The model under review builds one solid part; all positions refer to its coordinate system, in mm. A direction names the side the tool comes from. Give positions to 0.01 mm unless a question says otherwise; leave off trailing zeros. Write each loop counter-clockwise with the first axis right and the second up, starting at its lowest first coordinate (ties: lowest second). Pieces come first, ordered by that corner, then holes. Notation, with made-up numbers: (55.5, -1) -> (79.5, -1) arc R10 ccw to (79.5, 8) -> close; hole circle Ø4 at (-38.5, 20.5). An arc over 180 degrees is marked (long way). Use CSV: the item, a comma, the result in double quotes.
```python
from build123d import *

# Parameters (mm, degrees)
EXTRUDE_1_DEPTH = 5
SKETCH_2_R      = 11.25
EXTRUDE_2_DEPTH = 2
CHAMFER_1_SIZE  = 1.5
SKETCH_3_W      = 9.552486588
SKETCH_3_H      = 17
EXTRUDE_3_DEPTH = 9
FILLET_1_R      = 1
EXTRUDE_4_DEPTH = 2


with BuildPart() as part:
    # Эскиз1 → Бобышка-Вытянуть1 (new body)
    with BuildSketch(Plane(origin=(0, 0, 0), x_dir=(1, 0, 0), z_dir=(0, 1, 0))):
        with BuildLine():
            Line((-10.75, 1), (-9.698582371, 1))
            ThreePointArc((-9.698582371, 1), (9.75, 0), (-9.698582371, -1))
            Line((-9.698582371, -1), (-10.75, -1))
            Line((-10.75, -1), (-10.75, 1))
        make_face()
    extrude(amount=EXTRUDE_1_DEPTH)

    # Эскиз2 → Бобышка-Вытянуть2 (add)
    with BuildSketch(Plane(origin=(0, 5, 0), x_dir=(1, 0, 0), z_dir=(0, 1, 0))):
        Circle(SKETCH_2_R)
    extrude(amount=EXTRUDE_2_DEPTH)

    # Фаска1
    chamfer_1_edges = [part.edges().sort_by_distance(p)[0] for p in [
        (-11.25, 7, 0),
    ]]
    chamfer(chamfer_1_edges, length=CHAMFER_1_SIZE)

    # Эскиз3 → Бобышка-Вытянуть3 (add)
    with BuildSketch(Plane.XZ):
        Rectangle(SKETCH_3_W, SKETCH_3_H)
    extrude(amount=EXTRUDE_3_DEPTH)

    # Скругление1
    fillet_1_edges = [part.edges().sort_by_distance(p)[0] for p in [
        (-4.776243294, -4.5, 8.5),
        (-4.776243294, -4.5, -8.5),
        (4.776243294, -4.5, -8.5),
        (4.776243294, -4.5, 8.5),
    ]]
    fillet(fillet_1_edges, radius=FILLET_1_R)

    # Эскиз4 → Бобышка-Вытянуть4 (add, symmetric)
    with BuildSketch(Plane(origin=(0, 0, 0), x_dir=(0, 0, -1), z_dir=(1, 0, 0))):
        Polygon((-8.5, -9), (-13.010373574, 1.032772808), (-10.70938382, 4.9), (-9.85, 4.388668944), (-11.885037306, 0.968422681), (-7.587929745, -8.589966039), align=None)
        Polygon((11.885037306, 0.968422681), (7.587929745, -8.589966039), (8.5, -9), (13.010373574, 1.032772808), (10.70938382, 4.9), (9.85, 4.388668944), align=None)
    extrude(amount=EXTRUDE_4_DEPTH, both=True)


solid = part.part
```
Q1. To check wall thickness, follow probe 1 along Z at (x, y) = (1.5, 0.75); probe 2 along Z at (x, y) = (-3.25, -0.75); probe 3 along Y at (x, z) = (6, -6). State the ranges of each line that lie inside material, in increasing order.
Derived:
probe 1,"z = -12.88 to -11.79, -9.63 to 9.63, 11.79 to 12.88"
probe 2,"z = -8.5 to 8.5"
probe 3,"y = 0 to 7"
Q2. Consider section C-C (x = 0). Write out the cut boundary in (y, z), then the cut area to 3 significant figures.
Derived:
outline,"(-9, -8.5) -> (1.03, -13.01) -> (4.9, -10.71) -> (4.39, -9.85) -> (0.97, -11.89) -> (-6.56, -8.5) -> (0, -8.5) -> (0, -9.75) -> (5, -9.75) -> (5, -11.25) -> (5.5, -11.25) -> (7, -9.75) -> (7, 9.75) -> (5.5, 11.25) -> (5, 11.25) -> (5, 9.75) -> (0, 9.75) -> (0, 8.5) -> (-6.56, 8.5) -> (0.97, 11.89) -> (4.39, 9.85) -> (4.9, 10.71) -> (1.03, 13.01) -> (-9, 8.5) -> close"
area,"321 mm2"
Q3. Consider section B-B (y = 4). Write out the cut boundary in (x, z).
Derived:
outline,"(-10.75, -1) -> (-9.7, -1) arc R9.75 ccw (long way) to (-9.7, 1) -> (-10.75, 1) -> close; (-2, -11.24) -> (2, -11.24) -> (2, -10.08) -> (-2, -10.08) -> close; (-2, 10.08) -> (2, 10.08) -> (2, 11.24) -> (-2, 11.24) -> close"
Q4. Consider section D-D (y = -3). Write out the cut boundary in (x, z), then the cut area to 3 significant figures.
Derived:
outline,"(-4.78, -7.5) arc R1 ccw to (-3.78, -8.5) -> (3.78, -8.5) arc R1 ccw to (4.78, -7.5) -> (4.78, 7.5) arc R1 ccw to (3.78, 8.5) -> (-3.78, 8.5) arc R1 ccw to (-4.78, 7.5) -> close; (-2, -11.2) -> (2, -11.2) -> (2, -10.1) -> (-2, -10.1) -> close; (-2, 10.1) -> (2, 10.1) -> (2, 11.2) -> (-2, 11.2) -> close"
area,"170 mm2"
Q5. Machinability: for faces 5 (the flat face through (-4.776, -4, 0)), 6 (the flat face through (-2, -2, 11)), 7 (the flat face through (1, 5, 10)), 8 (the flat face through (-0.028, 2.702, 10.853)), which of the approach directions +Z, -Z, +X, -X, +Y, -Y give a long, thin tool a straight path to every point of the face, cutting with its end or side? Answer none if there is none.
Derived:
face 5,"+Z, -Z, -X, -Y"
face 6,"+Z, -X, -Y"
face 7,"none"
face 8,"+X, -X"
Q6. Consider section A-A (z = 0). Write out the cut boundary in (x, y), then the cut area to 3 significant figures.
Derived:
outline,"(-11.25, 5) -> (-10.75, 5) -> (-10.75, 0) -> (-4.78, 0) -> (-4.78, -9) -> (4.78, -9) -> (4.78, 0) -> (9.75, 0) -> (9.75, 5) -> (11.25, 5) -> (11.25, 5.5) -> (9.75, 7) -> (-9.75, 7) -> (-11.25, 5.5) -> close"
area,"231 mm2"
Q7. The part is to be moulded in two halves that separate along Z. For faces 1 (the cylindrical face through (4.48, -4.56, -8.21)), 2 (the cylindrical face through (-4.49, -4.56, 8.2)), 3 (the cylindrical face through (5.19, 5.25, 9.98)), 4 (the flat face through (-0.03, 4.65, 10.29)), say which applies: pulls with the +Z half, pulls with the -Z half, needs draft (parallel to the pull), parting line crosses it, or undercut.
Derived:
face 1,"pulls with the -Z half"
face 2,"pulls with the +Z half"
face 3,"parting line crosses it"
face 4,"undercut"
Q8. Insertion check: pin 1 (7 mm diameter, centred on y = -6.5, z = 3, fed in from -X); pin 2 (4 mm diameter, centred on x = -1.5, y = -5.5, fed in from -Z); pin 3 (6 mm diameter, centred on x = -1, y = -6, fed in from -Z). Each pin has a flat end and moves straight along its axis. Give the tip position at first contact, or say it passes through.
Derived:
pin 1,"stops at x = -4.78"
pin 2,"stops at z = -10.97"
pin 3,"stops at z = -11.2"
